Geometry: final body of the model. Coordinates: model frame, mm. Face numbers are marked on the shaded views. A direction names the side the tool comes from. Round coordinates to 2 decimals unless told otherwise and drop trailing zeros. Loops run counter-clockwise (first coordinate to the right, second up) from the corner with the lowest first, then second, coordinate; pieces in that order, holes last. Notation, with made-up numbers: (-26.75, 8) - (32.25, 8) arc R30 cw to (32.25, 31) - close; hole circle Ø7 at (36, 41). An arc over 180 degrees is marked (long way). Answer as a JSON object with one key per item and string values. Group by question number.
Item 1: Line query: line 1 (Z direction, x = 238.5, y = 25); line 2 (Y direction, x = 140, z = 89); line 3 (X direction, y = -124, z = 6.5). Output: solid intervals per line, ascending.
Item 2: Section A-A (y = 0). Return the cut outline in (x, z), plus the area to 3 significant figures.
Item 3: Section C-C (z = 82.5). Return the cut outline in (x, y).
Item 4: Section D-D (x = 181.5). Return the cut outline in (y, z).
Item 5: Section B-B (y = 138.5). Return the cut outline in (x, z).
Item 6: First-contact query: pin 1 (2 mm diameter, centred on x = 185, y = 108.5, fed in from +Z); pin 2 (2 mm diameter, centred on y = -41, z = 44, fed in from +X); pin 3 (21.5 mm diameter, centred on x = 120.1, y = -131.21, fed in from +Z). Flat tips, straight axial feed; report the tip coordinate or a pass-through.
Item 7: Draft query along Y for the marked faces 3, 4 and 5. Return one class per face: released by +Y, released by -Y, zero draft, split by the parting line, or undercut.
Item 8: Reachability of the marked faces 1 and 2 from +Z, -Z, +X, -X, +Y, -Y: full face, straight path, thin tool, end or side. Return the list, or none.
```python
from build123d import *

# Parameters (mm, degrees)
SKETCH1_W           = 320
SKETCH1_H           = 320
BOSS_EXTRUDE1_DEPTH = 20
SKETCH2_R           = 105
SKETCH2_R_2         = 100
BOSS_EXTRUDE2_DEPTH = 80
SKETCH4_R           = 12
CUT_EXTRUDE1_DEPTH  = 333.345210486


with BuildPart() as part:
    # Sketch1 → Boss-Extrude1 (new body)
    with BuildSketch(Plane.XY):
        with Locations((120.0952319, 0)):
            Rectangle(SKETCH1_W, SKETCH1_H)
    extrude(amount=BOSS_EXTRUDE1_DEPTH)

    # Sketch2 → Boss-Extrude2 (add)
    with BuildSketch(Plane.XY.offset(20)):
        with Locations(Location((120.0952319, 0, 0), (0, 0, 180))):
            Circle(SKETCH2_R)
        with Locations((120.0952319, 0)):
            Circle(SKETCH2_R_2, mode=Mode.SUBTRACT)
    extrude(amount=BOSS_EXTRUDE2_DEPTH)

    # Sketch4 → Cut-Extrude1 (cut, through all)
    with BuildSketch(Plane.XY.offset(20)):
        with Locations((120.0952319, 131.208738881)):
            Circle(SKETCH4_R)
        with Locations((251.303970781, 0)):
            Circle(SKETCH4_R)
        with Locations((120.0952319, -131.208738881)):
            Circle(SKETCH4_R)
        with Locations((-11.113506981, 0)):
            Circle(SKETCH4_R)
    extrude(amount=-CUT_EXTRUDE1_DEPTH, mode=Mode.SUBTRACT)


solid = part.part
```
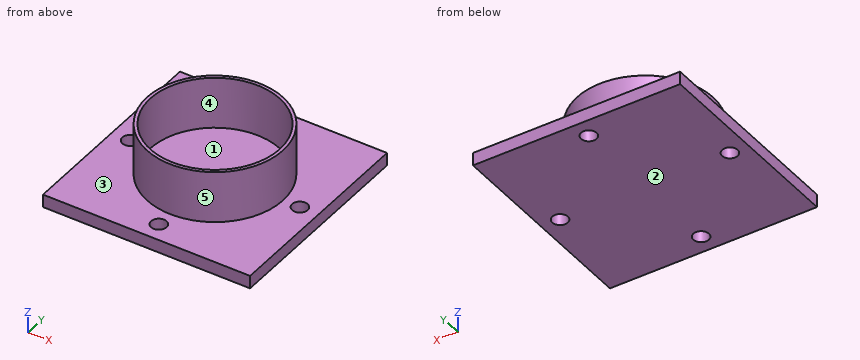
Values:
{
 "1": {"line 1": "z = 0 to 20", "line 2": "y = -103.1 to -98, 98 to 103.1", "line 3": "x = -39.9 to 110.5, 129.69 to 280.1"},
 "2": {"outline": "(-39.9, 0) - (-23.11, 0) - (-23.11, 20) - (-39.9, 20) - close; (0.89, 0) - (239.3, 0) - (239.3, 20) - (225.1, 20) - (225.1, 100) - (220.1, 100) - (220.1, 20) - (20.1, 20) - (20.1, 100) - (15.1, 100) - (15.1, 20) - (0.89, 20) - close; (263.3, 0) - (280.1, 0) - (280.1, 20) - (263.3, 20) - close", "area": "6,240 mm^2"},
 "3": {"outline": "circle Ø210 at (120.1, 0); hole circle Ø200 at (120.1, 0)"},
 "4": {"outline": "(-160, 0) - (160, 0) - (160, 20) - (85.17, 20) - (85.17, 100) - (78.93, 100) - (78.93, 20) - (-78.93, 20) - (-78.93, 100) - (-85.17, 100) - (-85.17, 20) - (-160, 20) - close"},
 "5": {"outline": "(-39.9, 0) - (110.56, 0) - (110.56, 20) - (-39.9, 20) - close; (129.63, 0) - (280.1, 0) - (280.1, 20) - (129.63, 20) - close"},
 "6": {"pin 1": "stops at z = 20", "pin 2": "stops at x = 217.18", "pin 3": "passes through"},
 "7": {"face 3": "zero draft", "face 4": "undercut", "face 5": "split by the parting line"},
 "8": {"face 1": "+Z", "face 2": "-Z, +X, -X, +Y, -Y"}
}
